from build123d import *

# Parameters (mm, degrees)
SKETCH1_W           = 88.9
SKETCH1_H           = 88.9
BOSS_EXTRUDE1_DEPTH = 10
CUT_EXTRUDE1_REACH  = 12
SKETCH2_W           = 50.8
SKETCH2_H           = 50.8


with BuildPart() as part:
    # Sketch1 → Boss-Extrude1 (new body)
    with BuildSketch(Plane(origin=(0, 0, 0), x_dir=(1, 0, 0), z_dir=(0, 1, 0))):
        Rectangle(SKETCH1_W, SKETCH1_H)
    extrude(amount=BOSS_EXTRUDE1_DEPTH)

    # Sketch2 → Cut-Extrude1 (cut, up to next)
    with BuildSketch(Plane(origin=(0, 10, 0), x_dir=(1, 0, 0), z_dir=(0, 1, 0)), mode=Mode.PRIVATE) as cut_extrude1_sk1:
        Rectangle(SKETCH2_W, SKETCH2_H)
    cut_extrude1_tool1 = extrude(cut_extrude1_sk1.sketch, amount=-CUT_EXTRUDE1_REACH, mode=Mode.PRIVATE) & part.part
    add(cut_extrude1_tool1.solids().sort_by_distance((0, 10, 0))[0], mode=Mode.SUBTRACT)


solid = part.part
Here's how the part is built. I have some questions about the finished solid (model axes, mm). A direction names the side the tool comes from. Round coordinates to 2 decimals unless told otherwise and drop trailing zeros. Order: outer loops, then holes, each group sorted by start corner. A loop starts at its lowest first (then second) coordinate and runs counter-clockwise, first axis right, second up. Notation, with made-up numbers: M 19.25,-20.75 L 61.25,-20.75 A17 cw 61.25,-1.75 Z; hole C 82,18.25 d2. An arc over 180 degrees is marked long. Return JSON: item names as keys, results as strings. Group by question number.
1. If we section it at B-B on x = -17: List the corners of the cut face in (y, z) for me, then the cut area to 3 significant figures.
2. On a 3-axis mill with a long thin cutter (end or side, diameter ignored), from which of +Z, -Z, +X, -X, +Y, -Y can I reach the whole of each face in a straight line? I mean faces 1 (the face through (44.45, 5, 1)), 2 (the face through (0, 5, -25.4)). Say none if no direction works.
3. If we mould it in two halves opening along Z, with no side actions, what happens to faces 3 (the face through (-1, 5, -44.45)), 4 (the face through (-25.4, 5, 0)), 5 (the face through (-1, 10, 29))? For each: pulls with the +Z half, pulls with the -Z half, needs draft (parallel to the pull), parting line crosses it, or undercut.
4. If we section it at A-A on z = 11.5: List the corners of the cut face in (x, y) for me.
5. If we section it at C-C on y = 7.75: List the corners of the cut face in (x, z) for me.
6. I'm going to push a flat-ended pin straight in: pin 1 Ø10 at (x, z) = (-22.5, 24.5) entering from -Y. Where does the tip first touch, or does it pass through?
7. Please list where this line runs through material, in increasing order: probe 1 along Z at (x, y) = (4, 9).
Reply:
{
 "1": {"outline": "M 0,-44.45 L 10,-44.45 L 10,-25.4 L 0,-25.4 Z; M 0,25.4 L 10,25.4 L 10,44.45 L 0,44.45 Z", "area": "381 mm^2"},
 "2": {"face 1": "+Z, -Z, +X, +Y, -Y", "face 2": "+Y, -Y"},
 "3": {"face 3": "pulls with the -Z half", "face 4": "undercut", "face 5": "needs draft"},
 "4": {"outline": "M -44.45,0 L -25.4,0 L -25.4,10 L -44.45,10 Z; M 25.4,0 L 44.45,0 L 44.45,10 L 25.4,10 Z"},
 "5": {"outline": "M -44.45,-44.45 L 44.45,-44.45 L 44.45,44.45 L -44.45,44.45 Z; hole M -25.4,-25.4 L 25.4,-25.4 L 25.4,25.4 L -25.4,25.4 Z"},
 "6": {"pin 1": "y = 0"},
 "7": {"probe 1": "-44.45 to -25.4, 25.4 to 44.45"}
}
